Could you check a few things on this model? Use its own coordinates, in mm. Face numbers are marked on the shaded views. A direction names the side the tool comes from. Coordinates: 2 decimals unless noted, no trailing zeros. Write each loop counter-clockwise with the first axis right and the second up, starting at its lowest first coordinate (ties: lowest second). Pieces come first, ordered by that corner, then holes. Notation, with made-up numbers: (40.25, 13.25) - (86.25, 13.25) arc R38 cw to (86.25, 52.25) - close; hole circle Ø8 at (4, -14.75). An arc over 180 degrees is marked (long way). Write item = value, one per line. Start each with the question number.
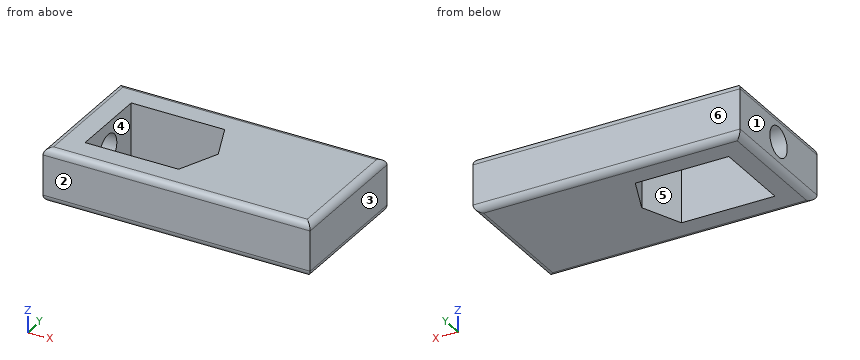
```python
from build123d import *

# Parameters (mm, degrees)
SKICA1_W                 = 40
SKICA1_H                 = 20
P_IDAT_VYSUNUT_M1_DEPTH  = 8
SKICA2_R                 = 2.25
ODEBRAT_VYSUNUT_M1_DEPTH = 8
ZAOBLIT2_R               = 1
ZAOBLIT3_R               = 1


with BuildPart() as part:
    # Skica1 → Přidat vysunutím1 (new body)
    with BuildSketch(Plane.XY):
        with Locations((20, 10)):
            Rectangle(SKICA1_W, SKICA1_H)
        Polygon((4, 16), (4, 4), (18, 4), (20.485281374, 10), (18, 16), align=None, mode=Mode.SUBTRACT)
    extrude(amount=P_IDAT_VYSUNUT_M1_DEPTH)

    # Skica2 → Odebrat vysunutím1 (cut)
    with BuildSketch(Plane.ZY):
        with Locations((4, 10)):
            Circle(SKICA2_R)
    extrude(amount=-ODEBRAT_VYSUNUT_M1_DEPTH, mode=Mode.SUBTRACT)

    # Zaoblit2
    zaoblit2_edges = [part.edges().sort_by_distance(p)[0] for p in [
        (20, 20, 8),
        (0, 10, 8),
        (20, 0, 8),
        (40, 10, 8),
    ]]
    fillet(zaoblit2_edges, radius=ZAOBLIT2_R)

    # Zaoblit3
    zaoblit3_edges = [part.edges().sort_by_distance(p)[0] for p in [
        (0, 10, 0),
        (20, 20, 0),
        (40, 10, 0),
        (20, 0, 0),
    ]]
    fillet(zaoblit3_edges, radius=ZAOBLIT3_R)


solid = part.part
```
1) Suppose I cut it at A-A on x = 17. Please give me the cut outline in (y, z), plus the area to 3 significant figures.
2) If I drill on probe 1 along Y at (x, z) = (2.7, 4); probe 2 along Y at (x, z) = (15, 3.25); probe 3 along X at (y, z) = (13.5, 6.5), over which ranges is the centre line in solid material (lowest first)? Write a range as [from, to].
3) Which directions (+Z, -Z, +X, -X, +Y, -Y) give clear straight access to the entire face, cutting with the end or side of a thin tool? Please do the marked faces 5 and 6.
4) Suppose I cut it at C-C on z = 4. Please give me the cut outline in (x, y).
5) Thinking about a two-plate mould opening in X: for the marked faces 1, 2, 3 and 4, which applies, +X half, -X half, draft (parallel to the pull), parting line (faces both ways), or undercut?
6) For P1, Ø4, axis at y = 10, z = 4, coming from the -X side; P2, Ø3, axis at x = 6, y = 9, coming from the +Z side; P3, Ø2.5, axis at x = 10, z = 4.5, coming from the -Y side, each with a flat end and sliding along its axis, tell me the tip position at first contact or that it passes through.
7) Suppose I cut it at B-B on y = 6.5. Please give me the cut outline in (x, z).
Reply:
q1.outline = (0, 1) arc R1 ccw to (1, 0) - (4, 0) - (4, 8) - (1, 8) arc R1 ccw to (0, 7) - close; (16, 0) - (19, 0) arc R1 ccw to (20, 1) - (20, 7) arc R1 ccw to (19, 8) - (16, 8) - close
q1.area = 63.1 mm^2
q2.probe_1 = [0, 7.75], [12.25, 20]
q2.probe_2 = [0, 4], [16, 20]
q2.probe_3 = [0, 4], [19.04, 40]
q3.face_5 = +Z, -Z
q3.face_6 = +Z, -Z, +X, -X, +Y
q4.outline = (0, 0) - (40, 0) - (40, 20) - (0, 20) - (0, 12.25) - (4, 12.25) - (4, 16) - (18, 16) - (20.49, 10) - (18, 4) - (4, 4) - (4, 7.75) - (0, 7.75) - close
q5.face_1 = -X half
q5.face_2 = draft
q5.face_3 = +X half
q5.face_4 = undercut
q6.P1 = 19.66
q6.P2 = through
q6.P3 = 0
q7.outline = (0, 1) arc R1 ccw to (1, 0) - (4, 0) - (4, 8) - (1, 8) arc R1 ccw to (0, 7) - close; (19.04, 0) - (39, 0) arc R1 ccw to (40, 1) - (40, 7) arc R1 ccw to (39, 8) - (19.04, 8) - close
